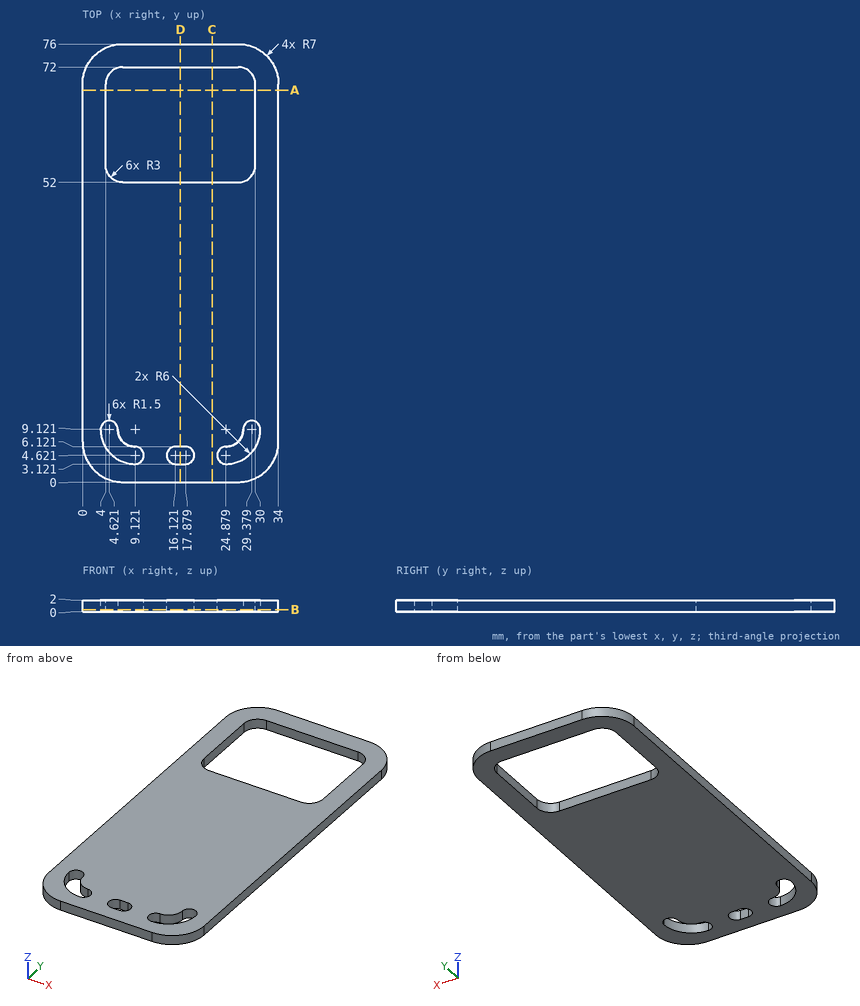
Part print with two shaded views. Sizes in mm from the minimum x, y, z corner. Coordinates: 2 decimals unless noted, no trailing zeros. Write each loop counter-clockwise with the first axis right and the second up, starting at its lowest first coordinate (ties: lowest second). Pieces come first, ordered by that corner, then holes. Notation, with made-up numbers: (74.5, -30.75) - (132.5, -30.75) arc R14 cw to (132.5, -19.75) - close; hole circle Ø10 at (78.25, 41). An arc over 180 degrees is marked (long way). One line per item, written item: value. Start each with the question number.
1. Probe line 1 (Y direction, x = 16.5, z = 0.2); line 2 (X direction, y = 66, z = 1.3); line 3 (Y direction, x = 27, z = 0.25). List the from-to ranges inside material, lowest first. Write a range as from..to.
2. Slice it at B-B (z = 0.35). Write the cut outline in (x, y).
3. Slice it at A-A (y = 68). Write the cut outline in (x, z).
4. Slice it at D-D (x = 17). Write the cut outline in (y, z), plus the area to 3 significant figures.
5. Slice it at C-C (x = 22.5). Write the cut outline in (y, z).
Answers below:
1. line 1: y = 0..3.12, 6.12..52, 72..76
1. line 2: x = 0..4, 30..34
1. line 3: y = 0..3.51, 7..52, 72..76
2. outline: (0, 7) arc R7 ccw to (7, 0) - (27, 0) arc R7 ccw to (34, 7) - (34, 69) arc R7 ccw to (27, 76) - (7, 76) arc R7 ccw to (0, 69) - close; hole (3.12, 9.12) arc R6 ccw to (9.12, 3.12) arc R1.5 ccw to (9.12, 6.12) arc R3 cw to (6.12, 9.12) arc R1.5 ccw to start; hole (4, 55) arc R3 ccw to (7, 52) - (27, 52) arc R3 ccw to (30, 55) - (30, 69) arc R3 ccw to (27, 72) - (7, 72) arc R3 ccw to (4, 69) - close; hole (16.12, 3.12) - (17.88, 3.12) arc R1.5 ccw to (17.88, 6.12) - (16.12, 6.12) arc R1.5 ccw to start; hole (24.88, 3.12) arc R6 ccw to (30.88, 9.12) arc R1.5 ccw to (27.88, 9.12) arc R3 cw to (24.88, 6.12) arc R1.5 ccw to start
3. outline: (0, 0) - (4, 0) - (4, 2) - (0, 2) - close; (30, 0) - (34, 0) - (34, 2) - (30, 2) - close
4. outline: (0, 0) - (3.12, 0) - (3.12, 2) - (0, 2) - close; (6.12, 0) - (52, 0) - (52, 2) - (6.12, 2) - close; (72, 0) - (76, 0) - (76, 2) - (72, 2) - close
4. area: 106 mm^2
5. outline: (0, 0) - (52, 0) - (52, 2) - (0, 2) - close; (72, 0) - (76, 0) - (76, 2) - (72, 2) - close
